The model under review builds one solid part; all positions refer to its coordinate system, in mm. Coordinates: 2 decimals unless noted, no trailing zeros. Loops run counter-clockwise (first coordinate to the right, second up) from the corner with the lowest first, then second, coordinate; pieces in that order, holes last. Notation, with made-up numbers: M 84,52.25 L 96,52.25 A22 ccw 96,60.25 Z; hole C 13,6 d10. An arc over 180 degrees is marked long. One line per item, written item: value.
Autodesk Inventor part; units mm, degrees
ref_plane "YZ Plane" through (0, 0, 0) normal (1, 0, 0) x (0, 1, 0)
ref_plane "XZ Plane" through (0, 0, 0) normal (0, 1, 0) x (-1, 0, 0)
ref_plane "XY Plane" through (0, 0, 0) normal (0, 0, 1) x (1, 0, 0)
sketch "Sketch1" plane through (0, 0, 0) normal (0, 0, 1) x (1, 0, 0)
  line L0 (3.6662, 6.35) -> (7.3323, 0)
  line L1 (7.3323, 0) -> (3.6662, -6.35)
  line L2 (3.6662, -6.35) -> (-3.6662, -6.35)
  line L3 (-3.6662, -6.35) -> (-7.3323, 0)
  line L4 (-7.3323, 0) -> (-3.6662, 6.35)
  line L5 (-3.6662, 6.35) -> (3.6662, 6.35)
  line L6 (0, 0) -> (0.4498, 0)
  dimension "d0" = 12.7
extrude "Extrusion1" add sketch "Sketch1" along normal blind 101.6
properties part number "Kermit HexShaft"
(1) Insertion check: pin 1 Ø2 at (x, y) = (-3.5, 0.5) entering from -Z; pin 2 Ø4 at (y, z) = (4.5, 54) entering from +X; pin 3 Ø6 at (y, z) = (-3.5, 45) entering from +X. Each pin has a flat end and moves straight along its axis. Give the tip position at first contact, or say it passes through.
Checks:
pin 1: z = 0
pin 2: x = 5.89
pin 3: x = 7.04
(2) To check wall thickness, follow L1, parallel to X at y = -1.5, z = 75; L2, parallel to X at y = -4.25, z = 72; L3, parallel to Y at x = -4, z = 93.5. State the ranges of each line that lie inside material, in increasing order. Write a range as [from, to].
Checks:
L1: [-6.47, 6.47]
L2: [-4.88, 4.88]
L3: [-5.77, 5.77]
(3) Add section A-A on z = 91. State the section outline as (x, y) points.
Checks:
outline: M -7.33,0 L -3.67,-6.35 L 3.67,-6.35 L 7.33,0 L 3.67,6.35 L -3.67,6.35 Z
(4) Add section C-C on x = 5. State the section outline as (y, z) points, then the cut area to 3 significant figures.
Checks:
outline: M -4.04,0 L 4.04,0 L 4.04,101.6 L -4.04,101.6 Z
area: 821 mm^2
(5) Add section B-B on y = 1.25. State the section outline as (x, z) points.
Checks:
outline: M -6.61,0 L 6.61,0 L 6.61,101.6 L -6.61,101.6 Z
